Verification items for the finished model (mm, model axes). A direction names the side the tool comes from. Round coordinates to 2 decimals unless told otherwise and drop trailing zeros. Order: outer loops, then holes, each group sorted by start corner. A loop starts at its lowest first (then second) coordinate and runs counter-clockwise, first axis right, second up. Notation, with made-up numbers: (39.25, 35) -> (96.25, 35) arc R11 cw to (96.25, 48) -> close; hole circle Ø5 at (61, 25.25). An arc over 180 degrees is marked (long way). Return JSON: item names as keys, results as strings. Group by question number.
Item 1: Sectioned sample at B-B on x = 330. Record the cut outline in (y, z), plus the area to 3 significant figures.
Item 2: Access from +Z, -Z, +X, -X, +Y, -Y to the whole of each face (thin tool, end or side, straight path). Record for faces 5 (the flat face through (-323, -50, -18)), 6 (the flat face through (323, -50, -18)), 7 (the cylindrical face through (-5.784, -294.943, -14.79)).
Item 3: Depth check by flat-ended pin: pin 1 Ø3 at (y, z) = (-159.5, -11) entering from -X; pin 2 Ø6 at (x, z) = (-206, -18) entering from +Y; pin 3 Ø5 at (y, z) = (-80.5, -25.5) entering from -X; pin 4 Ø11 at (x, z) = (330, -15) entering from -Y. Enter the tip coordinate at first touch or a pass-through.
Item 4: Sectioned sample at D-D on x = 0. Record the cut outline in (y, z), plus the area to 3 significant figures.
Item 5: Sectioned sample at C-C on y = -154. Record the cut outline in (x, z).
Item 6: Sectioned sample at A-A on z = -15. Record the cut outline in (x, y).
Item 7: Draft check along Z on faces 1 (the cylindrical face through (336.834, -24.65, -13.483)), 2 (the flat face through (-28, -245, -30)), 3 (the flat face through (-28, -245, 0)), 4 (the cylindrical face through (-5.168, -234.943, -14.79)). Enter one of: pulls with the +Z half, pulls with the -Z half, needs draft (parallel to the pull), parting line crosses it, or undercut.
Item 8: Scan lines: probe 1 along X at (y, z) = (-25, -18.5); probe 2 along X at (y, z) = (-24, -15); probe 3 along Z at (x, y) = (330, -31). Record each from-to range of solid material in increasing order. Write a range as from..to.
Autodesk Inventor part; units mm, degrees
ref_plane "YZ Plane" through (0, 0, 0) normal (1, 0, 0) x (0, 1, 0)
ref_plane "XZ Plane" through (0, 0, 0) normal (0, 1, 0) x (-1, 0, 0)
ref_plane "XY Plane" through (0, 0, 0) normal (0, 0, 1) x (1, 0, 0)
sketch "Sketch1" plane through (0, 0, 0) normal (0, 0, 1) x (1, 0, 0)
  circle A0 centre (0, 0) radius 265 construction
  line L0 (0, 265) -> (0, 295) construction
  line L1 (0, 265) -> (0, 235) construction
  circle A1 centre (0, 0) radius 235
  circle A2 centre (0, 0) radius 295
  line L2 (-235, 0) -> (-235, 80)
  line L3 (-235, 80) -> (-295, 80)
  line L4 (-295, 80) -> (-295, 0)
  line L5 (235, 0) -> (235, 80)
  line L6 (235, 80) -> (295, 80)
  line L7 (295, 80) -> (295, 0)
  line L8 (-235, 0) -> (-295, 0)
  line L9 (-295, 0) -> (-355, 0)
  line L10 (-355, 0) -> (-355, -50)
  line L11 (-355, -50) -> (-290.7318, -50)
  line L12 (235, 0) -> (295, 0)
  line L13 (295, 0) -> (355, 0)
  line L14 (355, 0) -> (355, -50)
  line L15 (355, -50) -> (290.7318, -50)
  dimension "d13" = 530
  dimension "d26" = 80
  dimension "d36" = 60
  dimension "d40" = 60
  dimension "d41" = 50
extrude "Extrusion1" add sketch "Sketch1" against normal blind 30 contours L12 A2 L8 A1 | L13 L14 L15 A2 | A2 L11 L10 L9
sketch "Sketch4" plane through (0, 0, 0) normal (0, 0, 1) x (1, 0, 0)
  line L0 (0, 0) -> (51.6989, -259.9081) construction
  line L1 (0, 0) -> (0, -276.8337) construction
  dimension "d27" = 265
  dimension "d35" = 11.25
sketch "Sketch7" plane through (0, 0, 0) normal (0, 0, 1) x (1, 0, 0)
  line L0 (-355, -50) -> (-355, 0) construction
  line L1 (-355, -25) -> (355, -25) construction
  line L2 (355, 0) -> (355, -50) construction
  point P0 (0, 0)
  point P1 (-330, -25)
  dimension "d42" = 25
fillet "Fillet2" [suppressed]
hole "Hole1" [suppressed]
hole "Hole2" [suppressed]
pattern_circular "Circular Pattern4" [suppressed]
sketch "Sketch8" plane through (-355, -50, -30) normal (0, -1, 0) x (1, 0, 0)
  line L0 (0, 30) -> (0, 0)
  point P0 (355, 30)
  point P1 (25, 15)
  point P2 (0, 15)
  dimension "d63" = 25
hole "Hole3" at (-330, -50, -15) direction (0, 1, 0) diameter 14 end through all
mirror "Mirror1" about plane through (0, 0, 0) normal (1, 0, 0) of "Hole3"
equation "\"d13\" = Шпил_пласт_КОРМА_диам_центров"
equation "\"d40\" = d36"
equation "\"d27\" = 0.5 * Шпил_пласт_КОРМА_диам_центров"
equation "\"BendReliefDepth\" = 0.5 * Thickness"
properties part number "Постель 201 зад_CPY"
Recorded:
{
 "1": {"outline": "(-50, -30) -> (0, -30) -> (0, -22) -> (-50, -22) -> close; (-50, -8) -> (0, -8) -> (0, 0) -> (-50, 0) -> close", "area": "800 mm²"},
 "2": {"face 5": "+Z, -Z, -X, -Y", "face 6": "+Z, -Z, +X, -Y", "face 7": "+Z, -Z, -Y"},
 "3": {"pin 1": "x = -249.12", "pin 2": "y = -107.44", "pin 3": "x = -284.5", "pin 4": "through"},
 "4": {"outline": "(-295, -30) -> (-235, -30) -> (-235, 0) -> (-295, 0) -> close", "area": "1,800 mm²"},
 "5": {"outline": "(-251.61, -30) -> (-177.51, -30) -> (-177.51, 0) -> (-251.61, 0) -> close; (177.51, -30) -> (251.61, -30) -> (251.61, 0) -> (177.51, 0) -> close"},
 "6": {"outline": "(-355, -50) -> (-337, -50) -> (-337, 0) -> (-355, 0) -> close; (-323, -50) -> (-290.73, -50) arc R295 ccw to (290.73, -50) -> (323, -50) -> (323, 0) -> (235, 0) arc R235 cw to (-235, 0) -> (-323, 0) -> close; (337, -50) -> (355, -50) -> (355, 0) -> (337, 0) -> close"},
 "7": {"face 1": "undercut", "face 2": "pulls with the -Z half", "face 3": "pulls with the +Z half", "face 4": "needs draft"},
 "8": {"probe 1": "-355..-336.06, -323.94..-233.67, 233.67..323.94, 336.06..355", "probe 2": "-355..-337, -323..-233.77, 233.77..323, 337..355", "probe 3": "-30..-22, -8..0"}
}
